Read the model definition and answer for the solid it produces. Units are mm, in the model's axes. Coordinates: 2 decimals unless noted, no trailing zeros. Write each loop counter-clockwise with the first axis right and the second up, starting at its lowest first coordinate (ties: lowest second). Pieces come first, ordered by that corner, then holes.
(1) Straight lines are drawn through the part: line 1 along Y through (x, z) = (-1.75, 8.5); line 2 along X through (y, z) = (-2.25, 4.25) (3 decimals); line 3 along Y through (x, z) = (-2.05, 5.25). For each, find the intervals that lie inside material, in ascending order.
(2) Given pin 1 (1 mm diameter, centred on x = 1, z = 7.5, fed in from +Y), flat-ended and moving along its own axis, determine where the tip first touches the part or whether it passes through.
(3) The part is cut by section B-B, the plane y = -0.8. Determine the outline of the cut face in (x, z), and give its area (3 significant figures).
(4) The part is cut by section A-A, the plane x = 0. Determine the outline of the cut face in (y, z), and give its area (3 significant figures).
```python
from build123d import *

# Parameters (mm, degrees)
BOSS_EXTRUDE1_DEPTH = 10
SKETCH2_R           = 2.55
CUT_EXTRUDE1_DEPTH  = 10


with BuildPart() as part:
    # Sketch1 → Boss-Extrude1 (new body)
    with BuildSketch(Plane.XY):
        with BuildLine():
            ThreePointArc((0.329389796, 2.981862231), (0.623735072, 2.934442802), (0.911920082, 2.858041596))
            ThreePointArc((0.911920082, 2.858041596), (1.086032069, 2.439267964), (1.513745185, 2.590091796))
            ThreePointArc((1.513745185, 2.590091796), (1.763355757, 2.427050983), (1.995550693, 2.240039605))
            ThreePointArc((1.995550693, 2.240039605), (1.984279326, 1.786653131), (2.436360281, 1.75047096))
            ThreePointArc((2.436360281, 1.75047096), (2.598076211, 1.5), (2.734132461, 1.234714416))
            ThreePointArc((2.734132461, 1.234714416), (2.539426662, 0.82510974), (2.93770655, 0.608177793))
            ThreePointArc((2.93770655, 0.608177793), (2.983565686, 0.31358539), (2.999957886, 0.015895887))
            ThreePointArc((2.999957886, 0.015895887), (2.655484058, -0.279102621), (2.931096668, -0.639274841))
            ThreePointArc((2.931096668, -0.639274841), (2.853169549, -0.927050983), (2.74706334, -1.205671185))
            ThreePointArc((2.74706334, -1.205671185), (2.312384136, -1.335055603), (2.417673544, -1.776191046))
            ThreePointArc((2.417673544, -1.776191046), (2.229434476, -2.007391819), (2.019176586, -2.218766755))
            ThreePointArc((2.019176586, -2.218766755), (1.569451989, -2.160165343), (1.486212701, -2.605987684))
            ThreePointArc((1.486212701, -2.605987684), (1.220209929, -2.740636373), (0.942155856, -2.848217397))
            ThreePointArc((0.942155856, -2.848217397), (0.555147336, -2.61176287), (0.29777218, -2.985185376))
            ThreePointArc((0.29777218, -2.985185376), (0, -3), (-0.29777218, -2.985185376))
            ThreePointArc((-0.29777218, -2.985185376), (-0.555147336, -2.61176287), (-0.942155856, -2.848217397))
            ThreePointArc((-0.942155856, -2.848217397), (-1.220209929, -2.740636373), (-1.486212701, -2.605987684))
            ThreePointArc((-1.486212701, -2.605987684), (-1.569451989, -2.160165343), (-2.019176586, -2.218766755))
            ThreePointArc((-2.019176586, -2.218766755), (-2.229434476, -2.007391819), (-2.417673544, -1.776191046))
            ThreePointArc((-2.417673544, -1.776191046), (-2.312384136, -1.335055603), (-2.74706334, -1.205671185))
            ThreePointArc((-2.74706334, -1.205671185), (-2.853169549, -0.927050983), (-2.931096668, -0.639274841))
            ThreePointArc((-2.931096668, -0.639274841), (-2.655484058, -0.279102621), (-2.999957886, 0.015895887))
            ThreePointArc((-2.999957886, 0.015895887), (-2.983565686, 0.31358539), (-2.93770655, 0.608177793))
            ThreePointArc((-2.93770655, 0.608177793), (-2.539426662, 0.82510974), (-2.734132461, 1.234714416))
            ThreePointArc((-2.734132461, 1.234714416), (-2.598076211, 1.5), (-2.436360281, 1.75047096))
            ThreePointArc((-2.436360281, 1.75047096), (-1.984279326, 1.786653131), (-1.995550693, 2.240039605))
            ThreePointArc((-1.995550693, 2.240039605), (-1.763355757, 2.427050983), (-1.513745185, 2.590091796))
            ThreePointArc((-1.513745185, 2.590091796), (-1.086032069, 2.439267964), (-0.911920082, 2.858041596))
            ThreePointArc((-0.911920082, 2.858041596), (-0.623735072, 2.934442802), (-0.329389796, 2.981862231))
            ThreePointArc((-0.329389796, 2.981862231), (0, 2.670111206), (0.329389796, 2.981862231))
        make_face()
    extrude(amount=BOSS_EXTRUDE1_DEPTH)

    # Sketch2 → Cut-Extrude1 (cut)
    with BuildSketch(Plane.XY.offset(10)):
        Circle(SKETCH2_R)
    extrude(amount=-CUT_EXTRUDE1_DEPTH, mode=Mode.SUBTRACT)


solid = part.part
```
Computed:
1. line 1: y = -2.1 to -1.85, 1.85 to 2.44
1. line 2: x = -1.485 to -1.2, 1.2 to 1.485
1. line 3: y = -2.19 to -1.52, 1.52 to 1.73
2. pin 1: stops at y = 2.96
3. outline: (-2.89, 0) - (-2.42, 0) - (-2.42, 10) - (-2.89, 10) - close; (2.42, 0) - (2.89, 0) - (2.89, 10) - (2.42, 10) - close
3. area: 9.40 mm2
4. outline: (-3, 0) - (-2.55, 0) - (-2.55, 10) - (-3, 10) - close; (2.55, 0) - (2.67, 0) - (2.67, 10) - (2.55, 10) - close
4. area: 5.70 mm2
